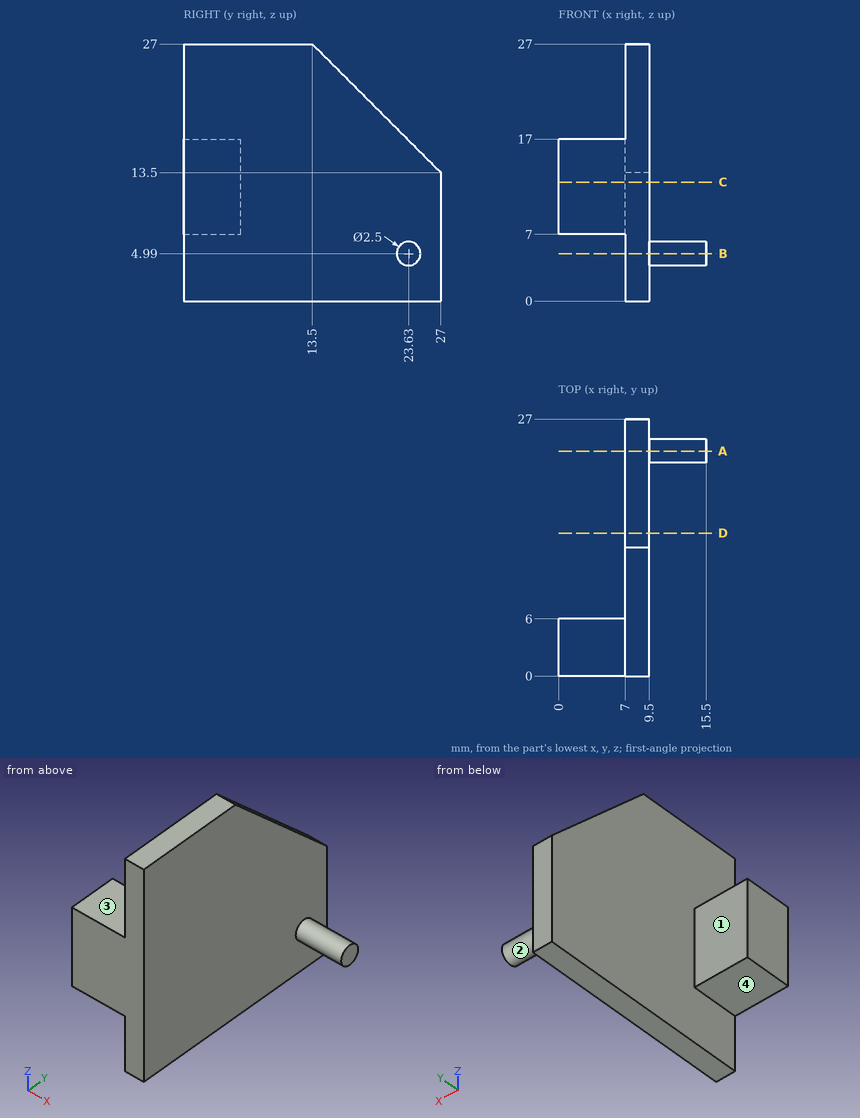
Geometry: see drawing. Coordinates: mm, zero at the bounding-box minimum. A direction names the side the tool comes from. Give positions to 0.01 mm unless a question says otherwise; leave off trailing zeros. Loops run counter-clockwise (first coordinate to the right, second up) from the corner with the lowest first, then second, coordinate; pieces in that order, holes last. Notation, with made-up numbers: (69.5, 72.5) -> (107.5, 72.5) arc R21 ccw to (107.5, 105.5) -> close; hole circle Ø4 at (-33, 2). An arc over 180 degrees is marked (long way). Use one line per item in the form item = value.
Item 1: Pin query (flat end, axial travel): P1, Ø12, axis at y = 13, z = 9, coming from the +X side; P2, Ø3.5, axis at x = 4, z = 10.5, coming from the +Y side; P3, Ø4, axis at y = 19.5, z = 9, coming from the -X side. Return the tip coordinate at first contact, or that it passes through.
A:
P1 = 9.5
P2 = 6
P3 = 7
Item 2: Section query C-C on z = 12.5. Output: boundary loops of the cut face in (x, y).
A:
outline = (0, 0) -> (9.5, 0) -> (9.5, 27) -> (7, 27) -> (7, 6) -> (0, 6) -> close
Item 3: Line query: probe 1 along X at (y, z) = (19.25, 11.25); probe 2 along X at (y, z) = (2, 12.5); probe 3 along Y at (x, z) = (6, 8.25). Output: solid intervals per line, ascending.
A:
probe_1 = 7 to 9.5
probe_2 = 0 to 9.5
probe_3 = 0 to 6
Item 4: Section query A-A on y = 23.63. Output: boundary loops of the cut face in (x, z), and give its area (3 significant figures).
A:
outline = (7, 0) -> (9.5, 0) -> (9.5, 3.74) -> (15.5, 3.74) -> (15.5, 6.24) -> (9.5, 6.24) -> (9.5, 16.87) -> (7, 16.87) -> close
area = 57.2 mm^2
Item 5: Section query B-B on z = 4.99. Output: boundary loops of the cut face in (x, y), and give its area (3 significant figures).
A:
outline = (7, 0) -> (9.5, 0) -> (9.5, 22.38) -> (15.5, 22.38) -> (15.5, 24.88) -> (9.5, 24.88) -> (9.5, 27) -> (7, 27) -> close
area = 82.5 mm^2
Item 6: Access query for the marked faces 1, 2, 3 and 4. Directions: +Z, -Z, +X, -X, +Y, -Y. A direction counts if a zero-diameter tool reaches every point of the face in a straight line with its end or side. Return the directions, or none.
A:
face_1 = +Z, -Z, -X, +Y
face_2 = +X
face_3 = +Z, -X, +Y, -Y
face_4 = -Z, -X, +Y, -Y
Item 7: Section query D-D on y = 15. Output: boundary loops of the cut face in (x, z).
A:
outline = (7, 0) -> (9.5, 0) -> (9.5, 25.5) -> (7, 25.5) -> close
